Design review of the part built by this model. Coordinates are the model's own, in mm. A direction names the side the tool comes from. Coordinates: 2 decimals unless noted, no trailing zeros. Loops run counter-clockwise (first coordinate to the right, second up) from the corner with the lowest first, then second, coordinate; pieces in that order, holes last. Notation, with made-up numbers: (-28.5, 68) -> (30.5, 68) arc R27 ccw to (30.5, 98) -> close; hole circle Ø10 at (36.25, 41.5). An arc over 180 degrees is marked (long way). Use a Markdown table: item, result. Add a question column.
Q1. Take a section at D-D on y = 38.5. Write out the cut boundary in (x, z).
Q2. Clearance check with flat-ended pins moving along their axes: pin 1 Ø2 at (x, z) = (32.5, 17) entering from -Y; pin 2 Ø4 at (y, z) = (-9.5, 4.5) entering from -X; pin 3 Ø3 at (x, y) = (33.5, 33) entering from +Z. State where each tip first meets the part, or that it passes through.
Q3. For faces 4 (the face through (50.7, -5.7, 7.5)), 5 (the face through (5.7, 45.7, 7.5)), 6 (the face through (45, -7, 4)), 7 (the face through (15, 47, 4)), 8 (the face through (30, 35, 24)), list the 3-axis set-ups (+Z, -Z, +X, -X, +Y, -Y) from which the entire face can be reached by the end or side of a thin tool; tool diameter is ignored.
Q4. For probe 1 along Y at (x, z) = (52.5, 3.5); probe 2 along Y at (x, z) = (7.5, 6.25); probe 3 along Z at (x, y) = (30, 27.5), list the stretches that pass through material, from the lowest coordinate up.
Q5. Take a section at A-A on y = -7.5. Write out the cut boundary in (x, z).
Q6. Draft analysis for pull direction Y (two halves, no side actions). For faces 1 (the face through (35, 23, 9.3)), 2 (the face through (52, -15, 4)), 3 (the face through (35, 8, 10)), state which applies: pulls with the +Y half, pulls with the -Y half, needs draft (parallel to the pull), parting line crosses it, or undercut.
Q7. Take a section at B-B on x = 7.5. Write out the cut boundary in (y, z).
Q8. Take a section at C-C on x = 56. Write out the cut boundary in (y, z).
from build123d import *

# Parameters (mm, degrees)
SKETCH1_W           = 60
SKETCH1_H           = 40
BOSS_EXTRUDE1_DEPTH = 40
SKETCH2_W           = 50
SKETCH2_H           = 30
CUT_EXTRUDE1_DEPTH  = 30
SKETCH3_W           = 50
SKETCH3_H           = 15.15
CUT_EXTRUDE2_DEPTH  = 0.7
SKETCH4_W           = 50
SKETCH4_H           = 10
CUT_EXTRUDE3_DEPTH  = 14
SKETCH5_W           = 41
SKETCH5_H           = 10
CUT_EXTRUDE4_DEPTH  = 2
SKETCH6_W           = 15
SKETCH6_H           = 7.5
BOSS_EXTRUDE3_DEPTH = 15
SKETCH7_W           = 15
SKETCH7_H           = 7.5
BOSS_EXTRUDE4_DEPTH = 15
CUT_EXTRUDE5_REACH  = 9.5
SKETCH8_R           = 2.25


with BuildPart() as part:
    # Sketch1 → Boss-Extrude1 (new body)
    with BuildSketch(Plane.XY):
        with Locations((30, 20)):
            Rectangle(SKETCH1_W, SKETCH1_H)
    extrude(amount=BOSS_EXTRUDE1_DEPTH)

    # Sketch2 → Cut-Extrude1 (cut)
    with BuildSketch(Plane.XY.offset(40)):
        with Locations((35, 15)):
            Rectangle(SKETCH2_W, SKETCH2_H)
    extrude(amount=-CUT_EXTRUDE1_DEPTH, mode=Mode.SUBTRACT)

    # Sketch3 → Cut-Extrude2 (cut)
    with BuildSketch(Plane.XY.offset(10)):
        with Locations((35, 22.425)):
            Rectangle(SKETCH3_W, SKETCH3_H)
    extrude(amount=-CUT_EXTRUDE2_DEPTH, mode=Mode.SUBTRACT)

    # Sketch4 → Cut-Extrude3 (cut)
    with BuildSketch(Plane.XY.offset(40)):
        with Locations((35, 35)):
            Rectangle(SKETCH4_W, SKETCH4_H)
    extrude(amount=-CUT_EXTRUDE3_DEPTH, mode=Mode.SUBTRACT)

    # Sketch5 → Cut-Extrude4 (cut)
    with BuildSketch(Plane.XY.offset(26)):
        with Locations((30.5, 35)):
            Rectangle(SKETCH5_W, SKETCH5_H)
    extrude(amount=-CUT_EXTRUDE4_DEPTH, mode=Mode.SUBTRACT)

    # Sketch6 → Boss-Extrude3 (add)
    with BuildSketch(Plane.XZ):
        with Locations((52.5, 3.75)):
            Rectangle(SKETCH6_W, SKETCH6_H)
    extrude(amount=BOSS_EXTRUDE3_DEPTH)

    # Sketch7 → Boss-Extrude4 (add)
    with BuildSketch(Plane(origin=(0, 40, 0), x_dir=(1, 0, 0), z_dir=(0, 1, 0))):
        with Locations((7.5, -3.75)):
            Rectangle(SKETCH7_W, SKETCH7_H)
    extrude(amount=BOSS_EXTRUDE4_DEPTH)

    # Sketch8 → Cut-Extrude5 (cut, up to next)
    with BuildSketch(Plane.XY.offset(7.5), mode=Mode.PRIVATE) as cut_extrude5_sk1:
        with Locations((52.5, -7.5)):
            Circle(SKETCH8_R)
    cut_extrude5_tool1 = extrude(cut_extrude5_sk1.sketch, amount=-CUT_EXTRUDE5_REACH, mode=Mode.PRIVATE) & part.part
    add(cut_extrude5_tool1.solids().sort_by_distance((52.5, -7.5, 7.5))[0], mode=Mode.SUBTRACT)
    # Sketch8 → Cut-Extrude5 (cut, up to next)
    with BuildSketch(Plane.XY.offset(7.5), mode=Mode.PRIVATE) as cut_extrude5_sk2:
        with Locations((7.5, 47.5)):
            Circle(SKETCH8_R)
    cut_extrude5_tool2 = extrude(cut_extrude5_sk2.sketch, amount=-CUT_EXTRUDE5_REACH, mode=Mode.PRIVATE) & part.part
    add(cut_extrude5_tool2.solids().sort_by_distance((7.5, 47.5, 7.5))[0], mode=Mode.SUBTRACT)


solid = part.part
Answer list:
| question | item | result |
|---|---|---|
| 1 | outline | (0, 0) -> (60, 0) -> (60, 26) -> (51, 26) -> (51, 24) -> (10, 24) -> (10, 40) -> (0, 40) -> close |
| 2 | pin 1 | y = 30 |
| 2 | pin 2 | x = 45 |
| 2 | pin 3 | z = 24 |
| 3 | face 4 | +Z, +X, -X, -Y |
| 3 | face 5 | +Z, +X, -X, +Y |
| 3 | face 6 | +Z, -Z, -X, -Y |
| 3 | face 7 | +Z, -Z, +X, +Y |
| 3 | face 8 | +Z, +Y, -Y |
| 4 | probe 1 | -15 to -9.75, -5.25 to 40 |
| 4 | probe 2 | 0 to 45.25, 49.75 to 55 |
| 4 | probe 3 | 0 to 9.3 |
| 5 | outline | (45, 0) -> (50.25, 0) -> (50.25, 7.5) -> (45, 7.5) -> close; (54.75, 0) -> (60, 0) -> (60, 7.5) -> (54.75, 7.5) -> close |
| 6 | face 1 | undercut |
| 6 | face 2 | pulls with the -Y half |
| 6 | face 3 | needs draft |
| 7 | outline | (0, 0) -> (45.25, 0) -> (45.25, 7.5) -> (40, 7.5) -> (40, 40) -> (0, 40) -> close; (49.75, 0) -> (55, 0) -> (55, 7.5) -> (49.75, 7.5) -> close |
| 8 | outline | (-15, 0) -> (40, 0) -> (40, 26) -> (30, 26) -> (30, 9.3) -> (14.85, 9.3) -> (14.85, 10) -> (0, 10) -> (0, 7.5) -> (-15, 7.5) -> close |
